Design review of the part built by this model. Coordinates are the model's own, in mm. A direction names the side the tool comes from. Coordinates: 2 decimals unless noted, no trailing zeros. Write each loop counter-clockwise with the first axis right and the second up, starting at its lowest first coordinate (ties: lowest second). Pieces come first, ordered by that corner, then holes.
Q1. Take a section at D-D (y = 7). Give the boundary of the cut face in (x, z).
Q2. Take a section at A-A (x = -56.88). Give the boundary of the cut face in (y, z) (3 decimals).
Q3. Machinability: for faces 3 (the flat face through (-29, 0, 1.58)), 4 (the flat face through (-49, 1, 1.28)), which of the approach directions +Z, -Z, +X, -X, +Y, -Y give a long, thin tool a straight path to every point of the face, cutting with its end or side? Answer none if there is none.
Q4. Take a section at B-B (y = -3). Give the boundary of the cut face in (x, z), and give its area (3 significant figures).
Q5. Take a section at C-C (z = 0.4). Give the boundary of the cut face in (x, y) (3 decimals).
Q6. For probe 1 along Y at (x, z) = (-56.88, 0.6) (3 decimals); probe 2 along X at (y, z) = (-1.5, 0.65); probe 3 along X at (y, z) = (-2, 0.3), list the stretches that pass through material, from the lowest coordinate up.
Q7. Mouldability with a two-part tool opening along X and no side actions: class faces 1 (the cylindrical face through (0.86, 3.89, 0.78)), 2 (the flat face through (-29, 0, 0)) as pulls with the +X half, pulls with the -X half, needs draft (parallel to the pull), parting line crosses it, or undercut.
Q8. Insertion check: pin 1 (5 mm diameter, centred on x = -33.5, y = -3, fed in from -Z). The pin has a flat end and moves straight along its axis. Give the tip position at first contact, or say it passes through.
```python
from build123d import *

# Parameters (mm, degrees)
ESQUISSE1_R             = 3.985
BOSS_EXTRU_1_DEPTH      = 1.58
ENL_V_MAT_EXTRU_1_DEPTH = 0.3


with BuildPart() as part:
    # Esquisse1 → Boss.-Extru.1 (new body)
    with BuildSketch(Plane(origin=(0, 0, 0), x_dir=(0, 1, 0), z_dir=(0, 0, 1))):
        with BuildLine():
            ThreePointArc((-7.69243745, 1.754567206), (0, -7.89), (7.69243745, 1.754567206))
            ThreePointArc((7.69243745, 1.754567206), (4.687683834, 28.44), (7.69243745, 55.125432794))
            ThreePointArc((7.69243745, 55.125432794), (0, 64.77), (-7.69243745, 55.125432794))
            ThreePointArc((-7.69243745, 55.125432794), (-4.687683834, 28.44), (-7.69243745, 1.754567206))
        make_face()
        with Locations(Location((0, 0, 0), (0, 0, 90))):
            Circle(ESQUISSE1_R, mode=Mode.SUBTRACT)
        with Locations(Location((0, 56.88, 0), (0, 0, 90))):
            Circle(ESQUISSE1_R, mode=Mode.SUBTRACT)
    extrude(amount=BOSS_EXTRU_1_DEPTH)

    # Esquisse2 → Enlèv. mat.-Extru.1 (cut)
    with BuildSketch(Plane.XY.offset(1.58)):
        with BuildLine():
            Line((-46.465889749, 0.892630637), (-46.926526768, 0.45232615))
            add(Edge.make_bspline(
                [(-46.926526768, 0.45232615), (-46.965601753, 0.49272975), (-47.04192744, 0.571650638), (-47.164916845, 0.676134939), (-47.292821348, 0.763208466), (-47.423152822, 0.836541237), (-47.558255553, 0.892022704), (-47.696567385, 0.932452984), (-47.838971481, 0.957101797), (-47.935345095, 0.959922058), (-47.983818435, 0.961340573)],
                knots=[0, 0, 0, 0, 1.115251505, 2.178435587, 3.19620269, 4.182487026, 5.141301733, 6.088180966, 7.038406374, 8, 8, 8, 8], degree=3))
            add(Edge.make_bspline(
                [(-47.983818435, 0.961340573), (-48.024299564, 0.960219896), (-48.104184612, 0.958008364), (-48.221476797, 0.941795654), (-48.333672834, 0.914225235), (-48.441156787, 0.87622809), (-48.543612381, 0.827061802), (-48.641254426, 0.766764423), (-48.73384219, 0.695880524), (-48.820152642, 0.614776863), (-48.89910641, 0.526165019), (-48.968867091, 0.431616392), (-49.027302852, 0.331347589), (-49.075260131, 0.226374058), (-49.112616997, 0.11620993), (-49.139294493, 0.000929371), (-49.154724043, -0.119604909), (-49.157027007, -0.201543214), (-49.158197441, -0.243186671)],
                knots=[0, 0, 0, 0, 1.035432265, 2.043311493, 3.022114605, 3.98653278, 4.95457646, 5.923598177, 6.917315552, 7.932509744, 8.948865224, 9.949768934, 10.933144597, 11.912367597, 12.897413939, 13.903909035, 14.934704909, 16, 16, 16, 16], degree=3))
            add(Edge.make_bspline(
                [(-49.158197441, -0.243186671), (-49.157860135, -0.272414963), (-49.157195299, -0.330024526), (-49.149917488, -0.41524506), (-49.138198495, -0.497929125), (-49.12123821, -0.577951477), (-49.100029206, -0.655381463), (-49.075146216, -0.730887069), (-49.04393087, -0.803424977), (-49.009281366, -0.873837667), (-48.968984392, -0.940203842), (-48.925536819, -1.003489497), (-48.878425021, -1.063384413), (-48.82734385, -1.119643738), (-48.771574403, -1.171388264), (-48.712558114, -1.220174011), (-48.64929946, -1.264779706), (-48.583112483, -1.306324779), (-48.513425411, -1.342415337), (-48.442129016, -1.37510641), (-48.368142301, -1.401656422), (-48.292366099, -1.423058153), (-48.215071208, -1.44125713), (-48.13550161, -1.452462799), (-48.054347076, -1.460948721), (-47.999500233, -1.461472677), (-47.971899364, -1.46173635)],
                knots=[0, 0, 0, 0, 1.103660481, 2.175337485, 3.227646561, 4.255952547, 5.262355991, 6.258840057, 7.255597736, 8.242457506, 9.22035537, 10.185017736, 11.140346927, 12.096287581, 13.051739095, 14.01125915, 14.986044842, 15.97314143, 16.960198552, 17.947847494, 18.933482797, 19.925264591, 20.920966487, 21.929612487, 22.958107872, 24, 24, 24, 24], degree=3))
            add(Edge.make_bspline(
                [(-47.971899364, -1.46173635), (-47.925083547, -1.460382188), (-47.833102641, -1.457721612), (-47.698107435, -1.436916285), (-47.569470453, -1.4026927), (-47.46669012, -1.362276634), (-47.386164443, -1.322365244), (-47.324861437, -1.285449174), (-47.261469349, -1.244154496), (-47.197041071, -1.196922705), (-47.130851909, -1.144320601), (-47.064070258, -1.0851961), (-46.994986493, -1.021496087), (-46.949730403, -0.976032136), (-46.926526768, -0.952721927)],
                knots=[0, 0, 0, 0, 1.404581149, 2.759636711, 4.088442092, 5.392261763, 6.066678138, 6.783632037, 7.538459478, 8.336747902, 9.180226004, 10.074962426, 11.012997595, 12, 12, 12, 12], degree=3))
            Line((-46.926526768, -0.952721927), (-46.479912185, -1.421772408))
            add(Edge.make_bspline(
                [(-46.479912185, -1.421772408), (-46.511306786, -1.45208291), (-46.572582334, -1.511242527), (-46.665014796, -1.595243664), (-46.757330929, -1.670728023), (-46.847300567, -1.740435357), (-46.936397505, -1.80233492), (-47.024612296, -1.856488534), (-47.11094631, -1.90426582), (-47.197192299, -1.94486104), (-47.283886932, -1.979330597), (-47.373085521, -2.009006624), (-47.465060755, -2.034111475), (-47.560374377, -2.054367792), (-47.658137358, -2.070610624), (-47.759264632, -2.081574442), (-47.863115, -2.088945052), (-47.933558314, -2.089607362), (-47.969094877, -2.089941478)],
                knots=[0, 0, 0, 0, 1.244526981, 2.429050516, 3.560637417, 4.644440555, 5.67424972, 6.652764056, 7.595344123, 8.486817594, 9.369275933, 10.254498637, 11.166417451, 12.086725134, 13.032340136, 13.991389299, 14.986715468, 16, 16, 16, 16], degree=3))
            add(Edge.make_bspline(
                [(-47.969094877, -2.089941478), (-48.034371141, -2.088277456), (-48.162098645, -2.085021427), (-48.349279971, -2.060896459), (-48.527097207, -2.020451373), (-48.695982948, -1.963250867), (-48.855883492, -1.890179901), (-49.006757933, -1.800598328), (-49.148363093, -1.694744151), (-49.279555082, -1.573858086), (-49.39822448, -1.440349574), (-49.503114485, -1.29699806), (-49.589879501, -1.143099023), (-49.661922363, -0.980926042), (-49.718258934, -0.809739061), (-49.75791033, -0.629352906), (-49.782363056, -0.439941752), (-49.785038219, -0.310569568), (-49.786402569, -0.244588914)],
                knots=[0, 0, 0, 0, 1.078019885, 2.10938526, 3.111377082, 4.085535484, 5.04941344, 6.010039228, 6.978205633, 7.964457913, 8.951525778, 9.924444315, 10.892603023, 11.863865945, 12.85144698, 13.863884204, 14.910567087, 16, 16, 16, 16], degree=3))
            add(Edge.make_bspline(
                [(-49.786402569, -0.244588914), (-49.785826061, -0.201556895), (-49.784683562, -0.11627795), (-49.772675795, 0.009344844), (-49.755936269, 0.131804598), (-49.729380533, 0.249829774), (-49.697370213, 0.365010388), (-49.657561174, 0.476094562), (-49.610016997, 0.583401563), (-49.556270142, 0.687111029), (-49.495466864, 0.786543551), (-49.427542926, 0.880844849), (-49.354246958, 0.97074291), (-49.273817774, 1.05504507), (-49.187424118, 1.134491518), (-49.094675932, 1.20865172), (-48.99613105, 1.278589214), (-48.891522746, 1.342500485), (-48.782883283, 1.400311626), (-48.671582889, 1.451303521), (-48.557895017, 1.493921003), (-48.442300349, 1.529270632), (-48.324310499, 1.555656631), (-48.204767649, 1.57562998), (-48.082654633, 1.586795211), (-48.000666322, 1.58862303), (-47.959279172, 1.589545701)],
                knots=[0, 0, 0, 0, 1.071919942, 2.124283339, 3.142214191, 4.149696895, 5.136002878, 6.119640489, 7.086990633, 8.058538607, 9.028339693, 9.988281803, 10.952401235, 11.916291999, 12.888973767, 13.874849856, 14.873389453, 15.898127285, 16.927174885, 17.938320013, 18.946391617, 19.950418109, 20.947802303, 21.956882652, 22.968648068, 24, 24, 24, 24], degree=3))
            add(Edge.make_bspline(
                [(-47.959279172, 1.589545701), (-47.92397169, 1.589016803), (-47.853723825, 1.587964506), (-47.749112966, 1.579192466), (-47.645338735, 1.565416065), (-47.542772677, 1.54463041), (-47.440681134, 1.51995521), (-47.340405703, 1.487646441), (-47.240364486, 1.451632228), (-47.142126479, 1.408584591), (-47.045554557, 1.361594206), (-46.95291107, 1.308281908), (-46.862640542, 1.251928476), (-46.776743314, 1.189198667), (-46.693610345, 1.122367809), (-46.613676346, 1.051124096), (-46.537642783, 0.974279688), (-46.489928341, 0.919984577), (-46.465889749, 0.892630637)],
                knots=[0, 0, 0, 0, 0.996412454, 1.982464992, 2.961075852, 3.949442424, 4.934965278, 5.923860011, 6.921385422, 7.934793307, 8.949617135, 9.951082467, 10.950285876, 11.951772932, 12.951063433, 13.960125323, 14.972308753, 16, 16, 16, 16], degree=3))
        make_face()
    extrude(amount=-ENL_V_MAT_EXTRU_1_DEPTH, mode=Mode.SUBTRACT)


solid = part.part
```
Response:
1. outline: (-60.52, 0) - (-51.88, 0) - (-51.88, 1.58) - (-60.52, 1.58) - close; (-5, 0) - (3.64, 0) - (3.64, 1.58) - (-5, 1.58) - close
2. outline: (-7.89, 0) - (-3.985, 0) - (-3.985, 1.58) - (-7.89, 1.58) - close; (3.985, 0) - (7.89, 0) - (7.89, 1.58) - (3.985, 1.58) - close
3. face 3: +Z, +X, -X, +Y, -Y
3. face 4: +Z
4. outline: (-64.18, 0) - (-59.5, 0) - (-59.5, 1.58) - (-64.18, 1.58) - close; (-54.26, 0) - (-2.62, 0) - (-2.62, 1.58) - (-54.26, 1.58) - close; (2.62, 0) - (7.3, 0) - (7.3, 1.58) - (2.62, 1.58) - close
4. area: 96.4 mm2
5. outline: (-55.125, -7.692) arc R120 cw to (-1.755, -7.692) arc R7.89 ccw (long way) to (-1.755, 7.692) arc R120 cw to (-55.125, 7.692) arc R7.89 ccw (long way) to start; hole circle Ø7.97 at (-56.88, 0); hole circle Ø7.97 at (0, 0)
6. probe 1: y = -7.89 to -3.985, 3.985 to 7.89
6. probe 2: x = -64.63 to -60.57, -53.19 to -3.69, 3.69 to 7.75
6. probe 3: x = -64.51 to -60.33, -53.43 to -3.45, 3.45 to 7.63
7. face 1: undercut
7. face 2: needs draft
8. pin 1: stops at z = 0
